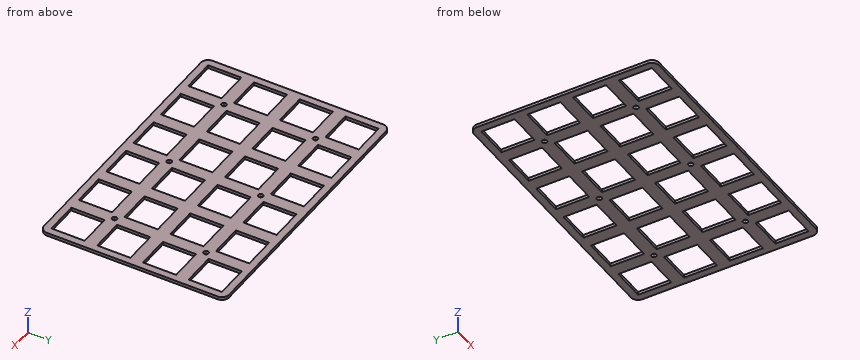
```python
from build123d import *

# Parameters (mm, degrees)
SKETCH_R  = 1
SKETCH_W  = 13.8
SKETCH_H  = 13.8
PAD_DEPTH = 1.3


with BuildPart() as part:
    # Sketch → Pad (new body)
    with BuildSketch(Plane.XY):
        with BuildLine():
            ThreePointArc((0, 16.8), (-2.12132, 15.92132), (-3, 13.8))
            Line((-3, 13.8), (-3, -57))
            ThreePointArc((-3, -57), (-2.12132, -59.12132), (0, -60))
            Line((0, -60), (108.8, -60))
            ThreePointArc((108.8, -60), (110.92132, -59.12132), (111.8, -57))
            Line((111.8, -57), (111.8, 13.8))
            ThreePointArc((111.8, 13.8), (110.92132, 15.92132), (108.8, 16.8))
            Line((108.8, 16.8), (0, 16.8))
        make_face()
        with Locations((92.4, -40.6)):
            Circle(SKETCH_R, mode=Mode.SUBTRACT)
        with Locations((54.4, -40.6)):
            Circle(SKETCH_R, mode=Mode.SUBTRACT)
        with Locations((16.4, -40.6)):
            Circle(SKETCH_R, mode=Mode.SUBTRACT)
        with Locations((16.4, -2.6)):
            Circle(SKETCH_R, mode=Mode.SUBTRACT)
        with Locations((54.4, -2.6)):
            Circle(SKETCH_R, mode=Mode.SUBTRACT)
        with Locations((92.4, -2.6)):
            Circle(SKETCH_R, mode=Mode.SUBTRACT)
        with Locations((6.9, 6.9)):
            Rectangle(SKETCH_W, SKETCH_H, mode=Mode.SUBTRACT)
        with Locations((25.9, 6.9)):
            Rectangle(SKETCH_W, SKETCH_H, mode=Mode.SUBTRACT)
        with Locations((44.9, 6.9)):
            Rectangle(SKETCH_W, SKETCH_H, mode=Mode.SUBTRACT)
        with Locations((63.9, 6.9)):
            Rectangle(SKETCH_W, SKETCH_H, mode=Mode.SUBTRACT)
        with Locations((82.9, 6.9)):
            Rectangle(SKETCH_W, SKETCH_H, mode=Mode.SUBTRACT)
        with Locations((101.9, 6.9)):
            Rectangle(SKETCH_W, SKETCH_H, mode=Mode.SUBTRACT)
        with Locations((6.9, -12.1)):
            Rectangle(SKETCH_W, SKETCH_H, mode=Mode.SUBTRACT)
        with Locations((25.9, -12.1)):
            Rectangle(SKETCH_W, SKETCH_H, mode=Mode.SUBTRACT)
        with Locations((44.9, -12.1)):
            Rectangle(SKETCH_W, SKETCH_H, mode=Mode.SUBTRACT)
        with Locations((63.9, -12.1)):
            Rectangle(SKETCH_W, SKETCH_H, mode=Mode.SUBTRACT)
        with Locations((82.9, -12.1)):
            Rectangle(SKETCH_W, SKETCH_H, mode=Mode.SUBTRACT)
        with Locations((101.9, -12.1)):
            Rectangle(SKETCH_W, SKETCH_H, mode=Mode.SUBTRACT)
        with Locations((6.9, -31.1)):
            Rectangle(SKETCH_W, SKETCH_H, mode=Mode.SUBTRACT)
        with Locations((25.9, -31.1)):
            Rectangle(SKETCH_W, SKETCH_H, mode=Mode.SUBTRACT)
        with Locations((44.9, -31.1)):
            Rectangle(SKETCH_W, SKETCH_H, mode=Mode.SUBTRACT)
        with Locations((63.9, -31.1)):
            Rectangle(SKETCH_W, SKETCH_H, mode=Mode.SUBTRACT)
        with Locations((82.9, -31.1)):
            Rectangle(SKETCH_W, SKETCH_H, mode=Mode.SUBTRACT)
        with Locations((101.9, -31.1)):
            Rectangle(SKETCH_W, SKETCH_H, mode=Mode.SUBTRACT)
        with Locations((6.9, -50.1)):
            Rectangle(SKETCH_W, SKETCH_H, mode=Mode.SUBTRACT)
        with Locations((25.9, -50.1)):
            Rectangle(SKETCH_W, SKETCH_H, mode=Mode.SUBTRACT)
        with Locations((44.9, -50.1)):
            Rectangle(SKETCH_W, SKETCH_H, mode=Mode.SUBTRACT)
        with Locations((63.9, -50.1)):
            Rectangle(SKETCH_W, SKETCH_H, mode=Mode.SUBTRACT)
        with Locations((82.9, -50.1)):
            Rectangle(SKETCH_W, SKETCH_H, mode=Mode.SUBTRACT)
        with Locations((101.9, -50.1)):
            Rectangle(SKETCH_W, SKETCH_H, mode=Mode.SUBTRACT)
    extrude(amount=PAD_DEPTH)


solid = part.part
```
Check sheet for the modelled part. Datum: model origin and axes. Units: mm. Give positions to 0.01 mm unless a question says otherwise; leave off trailing zeros. Write each loop counter-clockwise with the first axis right and the second up, starting at its lowest first coordinate (ties: lowest second). Pieces come first, ordered by that corner, then holes.
Item 1: Cross-section at C-C (z = 0.3). Count the separate pieces of the cut face and the enclosed holes in it, and give its area (3 significant figures).
Item 2: Cross-section at A-A (y = -9.5). Enter the section's corners in (x, z).
Item 3: Cross-section at B-B (x = 68.5). Enter the section's corners in (y, z).
Item 4: Scan lines: L1, parallel to Y at x = 92.5, z = 1.1; L2, parallel to Y at x = 12, z = 0.7; L3, parallel to Y at x = 93, z = 0.65. Record each from-to range of solid material in increasing order.
Report:
1. separate pieces: 1
1. enclosed holes: 30
1. area: 4,220 mm2
2. outline: (-3, 0) - (0, 0) - (0, 1.3) - (-3, 1.3) - close; (13.8, 0) - (19, 0) - (19, 1.3) - (13.8, 1.3) - close; (32.8, 0) - (38, 0) - (38, 1.3) - (32.8, 1.3) - close; (51.8, 0) - (57, 0) - (57, 1.3) - (51.8, 1.3) - close; (70.8, 0) - (76, 0) - (76, 1.3) - (70.8, 1.3) - close; (89.8, 0) - (95, 0) - (95, 1.3) - (89.8, 1.3) - close; (108.8, 0) - (111.8, 0) - (111.8, 1.3) - (108.8, 1.3) - close
3. outline: (-60, 0) - (-57, 0) - (-57, 1.3) - (-60, 1.3) - close; (-43.2, 0) - (-38, 0) - (-38, 1.3) - (-43.2, 1.3) - close; (-24.2, 0) - (-19, 0) - (-19, 1.3) - (-24.2, 1.3) - close; (-5.2, 0) - (0, 0) - (0, 1.3) - (-5.2, 1.3) - close; (13.8, 0) - (16.8, 0) - (16.8, 1.3) - (13.8, 1.3) - close
4. L1: y = -60 to -41.59, -39.61 to -3.59, -1.61 to 16.8
4. L2: y = -60 to -57, -43.2 to -38, -24.2 to -19, -5.2 to 0, 13.8 to 16.8
4. L3: y = -60 to -41.4, -39.8 to -3.4, -1.8 to 16.8
